from build123d import *

# Parameters (mm, degrees)
F1_DEPTH = 127
F3_DEPTH = 7.366


with BuildPart() as f1:
    # F0 (on Right) → F1 (new body)
    with BuildSketch(Plane.YZ):
        Polygon((0, -63.5), (0, 0), (-6.35, -10.998523), (-6.35, -63.5), align=None)
    extrude(amount=F1_DEPTH)

    # F2 (on Front) → F3 (cut)
    with BuildSketch(Plane.XZ):
        with BuildLine():
            Line((0, -44.45), (0, -33.842908))
            Line((0, -33.842908), (-28.897969, -33.245133))
            Line((-28.897969, -33.245133), (-28.897969, -77.647364))
            Line((-28.897969, -77.647364), (46.444243, -77.647364))
            Line((46.444243, -77.647364), (44.850173, -63.5))
            Line((44.850173, -63.5), (19.05, -63.5))
            ThreePointArc((19.05, -63.5), (5.579616, -57.920384), (0, -44.45))
        make_face()
        with BuildLine():
            Line((143.538471, -31.044858), (127, -30.048563))
            Line((127, -30.048563), (127, -44.45))
            ThreePointArc((127, -44.45), (121.420384, -57.920384), (107.95, -63.5))
            Line((107.95, -63.5), (99.701572, -63.5))
            Line((99.701572, -63.5), (99.701572, -83.425855))
            Line((99.701572, -83.425855), (143.538471, -83.425855))
            Line((143.538471, -83.425855), (143.538471, -31.044858))
        make_face()
    extrude(amount=F3_DEPTH, mode=Mode.SUBTRACT)


solid = f1.part
Work out the finished part from the listing and answer in its coordinate system (mm). Coordinates: 2 decimals unless noted, no trailing zeros. Loops run counter-clockwise (first coordinate to the right, second up) from the corner with the lowest first, then second, coordinate; pieces in that order, holes last. Notation, with made-up numbers: (-28.75, 75.25) -> (-17.75, 75.25) arc R14 ccw to (-17.75, 84.25) -> close; hole circle Ø8 at (53.5, 72). An arc over 180 degrees is marked (long way). Write each question's results on one line, items separated by ' | '. Start each with the question number.
1) Find section B-B on x = 67.5. Determine the outline of the cut face in (y, z), then the cut area to 3 significant figures.
2) Flat-ended cylindrical pins translate along their axes: P1, Ø1, axis at x = 113, y = -3.5, coming from the +Z side; P2, Ø1, axis at x = 55, z = -17, coming from the +Y side. Find the tip coordinate at first contact, or state that the pin passes through.
3) Consider line 1 along Z through (x, y) = (117, -6); line 2 along Z through (x, y) = (22, -5.5); line 3 along X through (y, z) = (-4, -56.5). Determine where each line is inside the solid, lowest interval first.
4) Find section C-C on z = -58. Determine the outline of the cut face in (x, y).
5) Find section A-A on y = -2.25. Determine the outline of the cut face in (x, z), then the cut area to 3 significant figures.
Response values:
1) outline: (-6.35, -63.5) -> (0, -63.5) -> (0, 0) -> (-6.35, -11) -> close | area: 368 mm^2
2) P1: stops at z = -5.2 | P2: stops at y = 0
3) line 1: z = -61.21 to -10.39 | line 2: z = -63.5 to -9.53 | line 3: x = 4.3 to 122.7
4) outline: (5.66, -6.35) -> (121.34, -6.35) -> (121.34, 0) -> (5.66, 0) -> close
5) outline: (0, -44.45) arc R19.05 ccw to (19.05, -63.5) -> (107.95, -63.5) arc R19.05 ccw to (127, -44.45) -> (127, -3.9) -> (0, -3.9) -> close | area: 7,410 mm^2
